The drawing under review shows one solid part. Ordinate dimensions are in mm from its lowest x, y, z. A direction names the side the tool comes from. Round coordinates to 2 decimals unless told otherwise and drop trailing zeros. Order: outer loops, then holes, each group sorted by start corner. A loop starts at its lowest first (then second) coordinate and runs counter-clockwise, first axis right, second up. Notation, with made-up numbers: M -18.5,-16.5 L 23.5,-16.5 A23 cw 23.5,-1.5 Z; hole C 9.5,-18 d2. An arc over 180 degrees is marked long. Answer as a JSON object with one key per item and string values. Group by question number.
1. Add section B-B on x = 13.1. State the section outline as (y, z) points.
2. To check wall thickness, follow probe 1 along X at (y, z) = (3.85, 7); probe 2 along Z at (x, y) = (13.1, 2.1); probe 3 along X at (y, z) = (4, 5.25). State the ranges of each line that lie inside material, in increasing order. Write a range as [from, to].
3. Mouldability with a two-part tool opening along X and no side actions: class the marked faces 1, 2, 3 and 4 as released by +X, released by -X, zero draft, split by the parting line, or undercut.
4. Add section D-D on x = 20. State the section outline as (y, z) points, and give its area (3 significant figures).
5. Machinability: for the marked faces 5 and 6, which of the approach directions +Z, -Z, +X, -X, +Y, -Y give a long, thin tool a straight path to every point of the face, cutting with its end or side? Answer none if there is none.
6. Clearance check with flat-ended pins moving along their axes: P1, Ø6, axis at y = 26.5, z = 8.5, coming from the -X side; P2, Ø6, axis at x = 16.5, z = 6, coming from the +Y side. State where each tip first meets the part, or that it passes through.
7. Add section A-A on z = 7. State the section outline as (x, y) points, and give its area (3 significant figures).
8. Add section C-C on z = 1.25. State the section outline as (x, y) points.
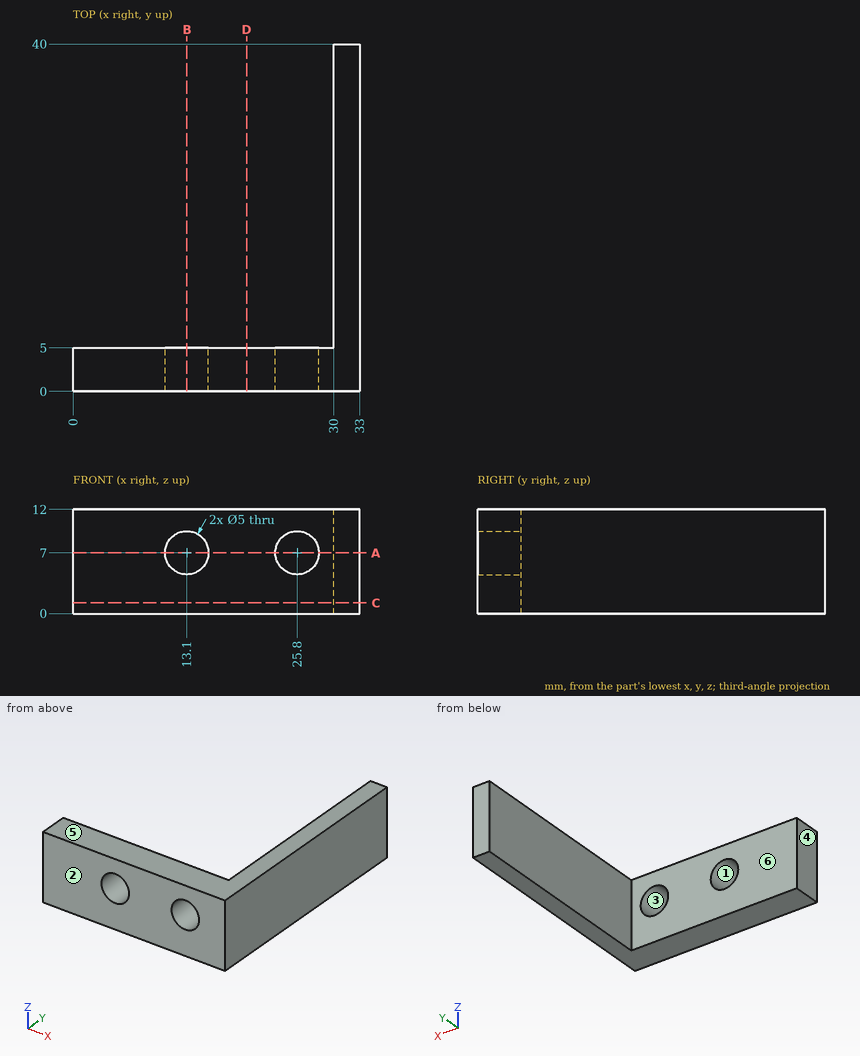
Recorded:
{
 "1": {"outline": "M 0,0 L 5,0 L 5,4.5 L 0,4.5 Z; M 0,9.5 L 5,9.5 L 5,12 L 0,12 Z"},
 "2": {"probe 1": "x = [0, 10.6], [15.6, 23.3], [28.3, 33]", "probe 2": "z = [0, 4.5], [9.5, 12]", "probe 3": "x = [0, 11.31], [14.89, 24.01], [27.59, 33]"},
 "3": {"face 1": "undercut", "face 2": "zero draft", "face 3": "undercut", "face 4": "released by -X"},
 "4": {"outline": "M 0,0 L 5,0 L 5,12 L 0,12 Z", "area": "60.0 mm²"},
 "5": {"face 5": "+Z, +X, -X, +Y, -Y", "face 6": "+Z, -Z, -X, +Y"},
 "6": {"P1": "stops at x = 30", "P2": "stops at y = 5"},
 "7": {"outline": "M 0,0 L 10.6,0 L 10.6,5 L 0,5 Z; M 15.6,0 L 23.3,0 L 23.3,5 L 15.6,5 Z; M 28.3,0 L 33,0 L 33,40 L 30,40 L 30,5 L 28.3,5 Z", "area": "220 mm²"},
 "8": {"outline": "M 0,0 L 33,0 L 33,40 L 30,40 L 30,5 L 0,5 Z"}
}
